Here's how the part is built. I have some questions about the finished solid (model axes, mm). Round coordinates to 2 decimals unless told otherwise and drop trailing zeros. Loops run counter-clockwise (first coordinate to the right, second up) from the corner with the lowest first, then second, coordinate; pieces in that order, holes last. Notation, with made-up numbers: (17, -38) -> (65, -38) arc R22 ccw to (65, -27) -> close; hole circle Ø1 at (75, 29). An arc over 180 degrees is marked (long way). Use one line per item in the form item = value. Start each with the question number.
Item 1: If we section it at A-A (x = 6): Write out the boundary of the cut face in (y, z).
Item 2: I'm going to push flat-ended pins straight in: pin 1 Ø2 at (y, z) = (13, 16) entering from +X; pin 2 Ø3 at (y, z) = (9, 14) entering from +X. Where does each tip first touch, or does it pass through?
Item 3: Thinking about a two-plate mould opening in Y: for faces 1 (the face through (7, 7, 0)), 2 (the face through (5.2, 11.4, 8.9)), 3 (the face through (13, 8, 14)), 4 (the face through (4, 18, 9)), which applies, released by +Y, released by -Y, zero draft, split by the parting line, or undercut?
Item 4: If we section it at B-B (z = 14): Write out the boundary of the cut face in (x, y), then the cut area to 3 significant figures.
Item 5: If we section it at D-D (y = 9.25): Write out the boundary of the cut face in (x, z).
Item 6: If we section it at C-C (y = 12): Write out the boundary of the cut face in (x, z), then the cut area to 3 significant figures.
Item 7: If I drill on L1, parallel to Z at x = 4, y = 9; L2, parallel to X at y = 5.5, z = 14; L3, parallel to Y at x = 6, z = 12.25, over which ranges is the centre line in solid material (lowest first)? Write a range as [from, to].
```python
from build123d import *

# Parameters (mm, degrees)
CYLINDER003_R          = 1
CYLINDER003_DEPTH      = 50
CYLINDER004_R          = 1
CYLINDER004_DEPTH      = 50
BOX002_W               = 18
BOX002_H               = 50
BOX002_DEPTH           = 18
BOX002_PLACEMENT_ANGLE = 45
CYLINDER002_R          = 1
CYLINDER002_DEPTH      = 50
ARRAY001_Y_COUNT       = 2
ARRAY001_Y_PITCH       = 8.485281
BOX001_W               = 18
BOX001_H               = 18
BOX001_DEPTH           = 18


with BuildPart() as cylinder003:
    # Cylinder003 → Cylinder003 (new body)
    with BuildSketch(Plane(origin=(-17, 9, 14), x_dir=(0, 0, -1), z_dir=(1, 0, 0))):
        Circle(CYLINDER003_R)
    extrude(amount=CYLINDER003_DEPTH)


with BuildPart() as cylinder004:
    # Cylinder004 → Cylinder004 (new body)
    with BuildSketch(Plane(origin=(9, 27, 14), x_dir=(1, 0, 0), z_dir=(0, -1, 0))):
        Circle(CYLINDER004_R)
    extrude(amount=CYLINDER004_DEPTH)


with BuildPart() as cube002:
    # Box002 → Box002 (new body)
    with BuildSketch(Plane.XY):
        with Locations((9, 25)):
            Rectangle(BOX002_W, BOX002_H)
    extrude(amount=BOX002_DEPTH)


with BuildPart() as cube002_1:
    # Box002 placement: moved
    add(cube002.part.moved(Location((28.8715, -3.57359, 0))).rotate(Axis((28.8715, -3.57359, 0), (0, 0, 1)), BOX002_PLACEMENT_ANGLE))


with BuildPart() as fusion001:
    # Cylinder002 → Cylinder002 (new body)
    with BuildSketch(Plane(origin=(6, 12, -10), x_dir=(1, 0, 0), z_dir=(0, 0, 1))):
        Circle(CYLINDER002_R)
    extrude(amount=CYLINDER002_DEPTH)

    # Array001 Y: Fusion001 ×2


with BuildPart() as fusion001_1:
    add(fusion001.part)
    with Locations(*[Vector(0.707107, -0.707107, 0) * (i * ARRAY001_Y_PITCH) for i in range(1, ARRAY001_Y_COUNT)]):
        add(fusion001.part)

    # Fusion001: union Cylinder003, Cylinder004, Cube002
    add(cylinder003.part)
    add(cylinder004.part)
    add(cube002_1.part)


with BuildPart() as cut001:
    # Box001 → Box001 (new body)
    with BuildSketch(Plane.XY):
        with Locations((9, 9)):
            Rectangle(BOX001_W, BOX001_H)
    extrude(amount=BOX001_DEPTH)

    # Cut001: cut Fusion001
    add(fusion001_1.part, mode=Mode.SUBTRACT)


solid = cut001.part
```
Values found:
q1.outline = (0, 0) -> (11, 0) -> (11, 18) -> (0, 18) -> close; (13, 0) -> (18, 0) -> (18, 18) -> (13, 18) -> close; hole circle Ø2 at (9, 14)
q2.pin_1 = 13.3
q2.pin_2 = 17.8
q3.face_1 = zero draft
q3.face_2 = undercut
q3.face_3 = undercut
q3.face_4 = released by +Y
q4.outline = (0, 0) -> (8, 0) -> (8, 8) -> (0, 8) -> close; (0, 10) -> (8, 10) -> (8, 17.3) -> (7.3, 18) -> (0, 18) -> close; (10, 0) -> (18, 0) -> (18, 7.3) -> (17.3, 8) -> (10, 8) -> close; (10, 10) -> (15.3, 10) -> (10, 15.3) -> close; hole circle Ø2 at (6, 12); hole circle Ø2 at (12, 6)
q4.area = 199 mm2
q5.outline = (0, 0) -> (16.05, 0) -> (16.05, 13.03) -> (9.25, 13.03) arc R1 cw to (8.75, 13.03) -> (0, 13.03) -> close; (0, 14.97) -> (8.75, 14.97) arc R1 cw to (9.25, 14.97) -> (16.05, 14.97) -> (16.05, 18) -> (0, 18) -> close
q6.outline = (0, 0) -> (5, 0) -> (5, 18) -> (0, 18) -> close; (7, 0) -> (13.3, 0) -> (13.3, 18) -> (7, 18) -> close; hole circle Ø2 at (9, 14)
q6.area = 200 mm2
q7.L1 = [0, 13], [15, 18]
q7.L2 = [0, 8], [10, 11.13], [12.87, 18]
q7.L3 = [0, 11], [13, 18]
